Part model, mm, in its own coordinate system. A direction names the side the tool comes from. Coordinates: 2 decimals unless noted, no trailing zeros. Order: outer loops, then holes, each group sorted by start corner. A loop starts at its lowest first (then second) coordinate and runs counter-clockwise, first axis right, second up.
from build123d import *

# Parameters (mm, degrees)
BASE_FLANGE1_DEPTH = 190
CUT_EXTRUDE1_REACH = 376.327
SKETCH6_R          = 55.1
SKETCH6_R_2        = 4.1
CUT_EXTRUDE2_REACH = 374.946
FILLET1_R          = 3
CUT_EXTRUDE3_REACH = 346.404
SKETCH8_R          = 3


# Sheet-metal steps are written as plain solids
with BuildPart() as part:
    # Sketch1 → Base-Flange1 (new body)
    with BuildSketch(Plane.XY):
        with BuildLine():
            Line((0, 0), (34, 0))
            ThreePointArc((34, 0), (34.707106781, 0.292893219), (35, 1))
            Line((35, 1), (35, 76))
            ThreePointArc((35, 76), (37.050252532, 80.949747468), (42, 83))
            Line((42, 83), (268, 83))
            ThreePointArc((268, 83), (272.949747468, 80.949747468), (275, 76))
            Line((275, 76), (275, 1))
            ThreePointArc((275, 1), (275.292893219, 0.292893219), (276, 0))
            Line((276, 0), (310, 0))
            Line((310, 0), (310, -6))
            Line((310, -6), (276, -6))
            ThreePointArc((276, -6), (271.050252532, -3.949747468), (269, 1))
            Line((269, 1), (269, 76))
            ThreePointArc((269, 76), (268.707106781, 76.707106781), (268, 77))
            Line((268, 77), (42, 77))
            ThreePointArc((42, 77), (41.292893219, 76.707106781), (41, 76))
            Line((41, 76), (41, 1))
            ThreePointArc((41, 1), (38.949747468, -3.949747468), (34, -6))
            Line((34, -6), (0, -6))
            Line((0, -6), (0, 0))
        make_face()
    extrude(amount=BASE_FLANGE1_DEPTH)

    # Sketch6 → Cut-Extrude1 (cut, up to next)
    with BuildSketch(Plane(origin=(0, 83, 0), x_dir=(1, 0, 0), z_dir=(0, 1, 0)), mode=Mode.PRIVATE) as cut_extrude1_sk1:
        with Locations(Location((155, -70, 0), (0, 0, 270))):
            Circle(SKETCH6_R)
    cut_extrude1_tool1 = extrude(cut_extrude1_sk1.sketch, amount=-CUT_EXTRUDE1_REACH, mode=Mode.PRIVATE) & part.part
    # Sketch6 → Cut-Extrude1 (cut, up to next)
    with BuildSketch(Plane(origin=(0, 83, 0), x_dir=(1, 0, 0), z_dir=(0, 1, 0)), mode=Mode.PRIVATE) as cut_extrude1_sk2:
        with Locations(Location((200.961940777, -24.038059223, 0), (0, 0, 270))):
            Circle(SKETCH6_R_2)
    cut_extrude1_tool2 = extrude(cut_extrude1_sk2.sketch, amount=-CUT_EXTRUDE1_REACH, mode=Mode.PRIVATE) & part.part
    # Sketch6 → Cut-Extrude1 (cut, up to next)
    with BuildSketch(Plane(origin=(0, 83, 0), x_dir=(1, 0, 0), z_dir=(0, 1, 0)), mode=Mode.PRIVATE) as cut_extrude1_sk3:
        with Locations(Location((200.961940777, -115.961940777, 0), (0, 0, 270))):
            Circle(SKETCH6_R_2)
    cut_extrude1_tool3 = extrude(cut_extrude1_sk3.sketch, amount=-CUT_EXTRUDE1_REACH, mode=Mode.PRIVATE) & part.part
    # Sketch6 → Cut-Extrude1 (cut, up to next)
    with BuildSketch(Plane(origin=(0, 83, 0), x_dir=(1, 0, 0), z_dir=(0, 1, 0)), mode=Mode.PRIVATE) as cut_extrude1_sk4:
        with Locations(Location((109.038059223, -24.038059223, 0), (0, 0, 270))):
            Circle(SKETCH6_R_2)
    cut_extrude1_tool4 = extrude(cut_extrude1_sk4.sketch, amount=-CUT_EXTRUDE1_REACH, mode=Mode.PRIVATE) & part.part
    # Sketch6 → Cut-Extrude1 (cut, up to next)
    with BuildSketch(Plane(origin=(0, 83, 0), x_dir=(1, 0, 0), z_dir=(0, 1, 0)), mode=Mode.PRIVATE) as cut_extrude1_sk5:
        with Locations(Location((109.038059223, -115.961940777, 0), (0, 0, 270))):
            Circle(SKETCH6_R_2)
    cut_extrude1_tool5 = extrude(cut_extrude1_sk5.sketch, amount=-CUT_EXTRUDE1_REACH, mode=Mode.PRIVATE) & part.part
    add(cut_extrude1_tool1.solids().sort_by_distance((155, 83, 70))[0], mode=Mode.SUBTRACT)
    add(cut_extrude1_tool2.solids().sort_by_distance((200.961941, 83, 24.038059))[0], mode=Mode.SUBTRACT)
    add(cut_extrude1_tool3.solids().sort_by_distance((200.961941, 83, 115.961941))[0], mode=Mode.SUBTRACT)
    add(cut_extrude1_tool4.solids().sort_by_distance((109.038059, 83, 24.038059))[0], mode=Mode.SUBTRACT)
    add(cut_extrude1_tool5.solids().sort_by_distance((109.038059, 83, 115.961941))[0], mode=Mode.SUBTRACT)

    # Sketch7 → Cut-Extrude2 (cut, up to next)
    with BuildSketch(Plane(origin=(0, 0, 0), x_dir=(1, 0, 0), z_dir=(0, 1, 0)), mode=Mode.PRIVATE) as cut_extrude2_sk1:
        with BuildLine():
            Line((299.5, -12), (299.5, -18))
            ThreePointArc((299.5, -18), (293, -24.5), (286.5, -18))
            Line((286.5, -18), (286.5, -12))
            ThreePointArc((286.5, -12), (293, -5.5), (299.5, -12))
        make_face()
    cut_extrude2_tool1 = extrude(cut_extrude2_sk1.sketch, amount=-CUT_EXTRUDE2_REACH, mode=Mode.PRIVATE) & part.part
    # Sketch7 → Cut-Extrude2 (cut, up to next)
    with BuildSketch(Plane(origin=(0, 0, 0), x_dir=(1, 0, 0), z_dir=(0, 1, 0)), mode=Mode.PRIVATE) as cut_extrude2_sk2:
        with BuildLine():
            Line((299.5, -178), (299.5, -172))
            ThreePointArc((299.5, -172), (293, -165.5), (286.5, -172))
            Line((286.5, -172), (286.5, -178))
            ThreePointArc((286.5, -178), (293, -184.5), (299.5, -178))
        make_face()
    cut_extrude2_tool2 = extrude(cut_extrude2_sk2.sketch, amount=-CUT_EXTRUDE2_REACH, mode=Mode.PRIVATE) & part.part
    # Sketch7 → Cut-Extrude2 (cut, up to next)
    with BuildSketch(Plane(origin=(0, 0, 0), x_dir=(1, 0, 0), z_dir=(0, 1, 0)), mode=Mode.PRIVATE) as cut_extrude2_sk3:
        with BuildLine():
            Line((10.5, -178), (10.5, -172))
            ThreePointArc((10.5, -172), (17, -165.5), (23.5, -172))
            Line((23.5, -172), (23.5, -178))
            ThreePointArc((23.5, -178), (17, -184.5), (10.5, -178))
        make_face()
    cut_extrude2_tool3 = extrude(cut_extrude2_sk3.sketch, amount=-CUT_EXTRUDE2_REACH, mode=Mode.PRIVATE) & part.part
    # Sketch7 → Cut-Extrude2 (cut, up to next)
    with BuildSketch(Plane(origin=(0, 0, 0), x_dir=(1, 0, 0), z_dir=(0, 1, 0)), mode=Mode.PRIVATE) as cut_extrude2_sk4:
        with BuildLine():
            Line((10.5, -12), (10.5, -18))
            ThreePointArc((10.5, -18), (17, -24.5), (23.5, -18))
            Line((23.5, -18), (23.5, -12))
            ThreePointArc((23.5, -12), (17, -5.5), (10.5, -12))
        make_face()
    cut_extrude2_tool4 = extrude(cut_extrude2_sk4.sketch, amount=-CUT_EXTRUDE2_REACH, mode=Mode.PRIVATE) & part.part
    add(cut_extrude2_tool1.solids().sort_by_distance((293, 0, 15))[0], mode=Mode.SUBTRACT)
    add(cut_extrude2_tool2.solids().sort_by_distance((293, 0, 175))[0], mode=Mode.SUBTRACT)
    add(cut_extrude2_tool3.solids().sort_by_distance((17, 0, 175))[0], mode=Mode.SUBTRACT)
    add(cut_extrude2_tool4.solids().sort_by_distance((17, 0, 15))[0], mode=Mode.SUBTRACT)

    # Fillet1
    fillet1_edges = [part.edges().sort_by_distance(p)[0] for p in [
        (0, -3, 0),
        (310, -3, 0),
        (0, -3, 190),
        (310, -3, 190),
    ]]
    fillet(fillet1_edges, radius=FILLET1_R)

    # Cut-Extrude3: up to this face of the body (flat: up to its plane)
    cut_extrude3_end = Plane(part.part.faces().sort_by_distance((35, 38.5, 95))[0])
    # Sketch8 → Cut-Extrude3 (cut, up to the picked face)
    with BuildSketch(Plane(origin=(275, 0, 0), x_dir=(0, 0, -1), z_dir=(1, 0, 0)), mode=Mode.PRIVATE) as cut_extrude3_sk1:
        with Locations((-172, 68.5)):
            Circle(SKETCH8_R)
    cut_extrude3_tool1 = split(extrude(cut_extrude3_sk1.sketch, amount=-CUT_EXTRUDE3_REACH, mode=Mode.PRIVATE), bisect_by=cut_extrude3_end, keep=Keep.BOTH, mode=Mode.PRIVATE)
    # Sketch8 → Cut-Extrude3 (cut, up to the picked face)
    with BuildSketch(Plane(origin=(275, 0, 0), x_dir=(0, 0, -1), z_dir=(1, 0, 0)), mode=Mode.PRIVATE) as cut_extrude3_sk2:
        with Locations((-172, 8.5)):
            Circle(SKETCH8_R)
    cut_extrude3_tool2 = split(extrude(cut_extrude3_sk2.sketch, amount=-CUT_EXTRUDE3_REACH, mode=Mode.PRIVATE), bisect_by=cut_extrude3_end, keep=Keep.BOTH, mode=Mode.PRIVATE)
    add(cut_extrude3_tool1.solids().sort_by(Axis((275, 68.5, 172), (-1, 0, 0)))[0], mode=Mode.SUBTRACT)
    add(cut_extrude3_tool2.solids().sort_by(Axis((275, 8.5, 172), (-1, 0, 0)))[0], mode=Mode.SUBTRACT)


solid = part.part
Q1. Cut at A-A on y = 68.5. Write the cut outline in (x, z), and give its area (3 significant figures).
Results list:
outline: (35, 0) - (41, 0) - (41, 169) - (35, 169) - close; (35, 175) - (41, 175) - (41, 190) - (35, 190) - close; (269, 0) - (275, 0) - (275, 169) - (269, 169) - close; (269, 175) - (275, 175) - (275, 190) - (269, 190) - close
area: 2,210 mm2
Q2. Cut at D-D on x = 172. Write the cut outline in (y, z), and give its area (3 significant figures).
Results list:
outline: (77, 0) - (83, 0) - (83, 17.59) - (77, 17.59) - close; (77, 122.41) - (83, 122.41) - (83, 190) - (77, 190) - close
area: 511 mm2
Q3. Mould opens along Z. For faces 6 (the face through (310, -3, 94)), 7 (the face through (156, 78, 190)), 8 (the face through (292.9, -3, 184.5)) say: pulls with the +Z half, pulls with the -Z half, needs draft (parallel to the pull), parting line crosses it, or undercut.
Results list:
face 6: needs draft
face 7: pulls with the +Z half
face 8: undercut
Q4. Pin check, flat tips, straight feed: pin 1 Ø10 at (y, z) = (14.5, 75.5) entering from +X; pin 2 Ø1 at (y, z) = (26, 98.5) entering from -X; pin 3 Ø12 at (x, z) = (115.5, 39.5) entering from -Y. Stop position of each tip, or through.
Results list:
pin 1: stops at x = 275
pin 2: stops at x = 35
pin 3: stops at y = 77
Q5. Which spindle directions (+Z, -Z, +X, -X, +Y, -Y) get a long thin tool onto all of the face, cutting with end or side? Do faces 1 (the face through (275, 39, 94)), 2 (the face through (38.042, 65.838, 170.616)), 3 (the face through (0, -3, 94)), 4 (the face through (10.5, -3, 15)), 5 (the face through (157, 77, 136)). Say none if no direction does.
Results list:
face 1: +Z, -Z, +X, +Y
face 2: +X, -X
face 3: +Z, -Z, -X, +Y, -Y
face 4: +Y, -Y
face 5: +Z, -Z, -Y
Q6. Wall check: line 1 along X through (y, z) = (32, 181); line 2 along Y through (x, z) = (270.2, 172); line 3 along Y through (x, z) = (272, 172). Give the ranges that are in metal, low to high.
Results list:
line 1: x = 35 to 41, 269 to 275
line 2: y = -2.92 to 5.5, 11.5 to 65.5, 71.5 to 82.65
line 3: y = -4.74 to 5.5, 11.5 to 65.5, 71.5 to 81.74
Q7. Cut at C-C on y = 51.5. Write the cut outline in (x, z).
Results list:
outline: (35, 0) - (41, 0) - (41, 190) - (35, 190) - close; (269, 0) - (275, 0) - (275, 190) - (269, 190) - close
Q8. Cut at B-B on x = 17. Write the cut outline in (y, z), and give its area (3 significant figures).
Results list:
outline: (-6, 0) - (0, 0) - (0, 5.5) - (-6, 5.5) - close; (-6, 24.5) - (0, 24.5) - (0, 165.5) - (-6, 165.5) - close; (-6, 184.5) - (0, 184.5) - (0, 190) - (-6, 190) - close
area: 912 mm2
